Here's how the part is built. I have some questions about the finished solid (model axes, mm). Face numbers are marked on the shaded views. A direction names the side the tool comes from. Give positions to 0.01 mm unless a question says otherwise; leave off trailing zeros. Loops run counter-clockwise (first coordinate to the right, second up) from the corner with the lowest first, then second, coordinate; pieces in that order, holes last. Notation, with made-up numbers: (19, -7.5) - (78, -7.5) arc R7 ccw to (78, 1.5) - close; hole circle Ø2 at (81.25, 71.25). An arc over 180 degrees is marked (long way). Use a Markdown table: item, result.
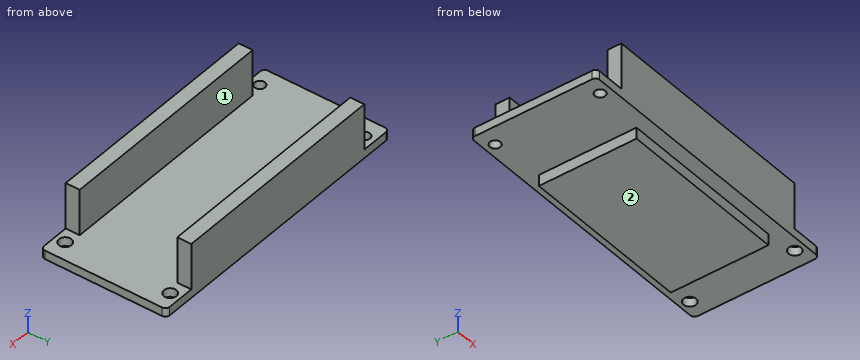
from build123d import *

# Parameters (mm, degrees)
SKETCH1_W           = 52.324
SKETCH1_H           = 22.86
BOSS_EXTRUDE1_DEPTH = 1.5748
SKETCH2_W           = 30.988
SKETCH2_H           = 17.78
BOSS_EXTRUDE2_DEPTH = 2.032
SKETCH3_W           = 40.64
SKETCH3_H           = 2.54
BOSS_EXTRUDE3_DEPTH = 8.382
FILLET1_R           = 0.762
SKETCH4_R           = 1.143
SKETCH4_R_2         = 0.9525
CUT_EXTRUDE1_DEPTH  = 1.5748


with BuildPart() as part:
    # Sketch1 → Boss-Extrude1 (new body)
    with BuildSketch(Plane.XY):
        with Locations((26.162, 11.43)):
            Rectangle(SKETCH1_W, SKETCH1_H)
    extrude(amount=BOSS_EXTRUDE1_DEPTH)

    # Sketch2 → Boss-Extrude2 (add)
    with BuildSketch(Plane(origin=(0, 0, 0), x_dir=(-1, 0, 0), z_dir=(0, 0, -1))):
        with Locations((-28.194, 11.43)):
            Rectangle(SKETCH2_W, SKETCH2_H)
    extrude(amount=BOSS_EXTRUDE2_DEPTH)

    # Sketch3 → Boss-Extrude3 (add)
    with BuildSketch(Plane.XY.offset(1.5748)):
        with Locations((26.162, 21.59)):
            Rectangle(SKETCH3_W, SKETCH3_H)
        with Locations((26.162, 1.27)):
            Rectangle(SKETCH3_W, SKETCH3_H)
    extrude(amount=BOSS_EXTRUDE3_DEPTH)

    # Fillet1
    fillet1_edges = [part.edges().sort_by_distance(p)[0] for p in [
        (0, 22.86, 0.7874),
        (52.324, 22.86, 0.7874),
        (52.324, 0, 0.7874),
        (0, 0, 0.7874),
    ]]
    fillet(fillet1_edges, radius=FILLET1_R)

    # Sketch4 → Cut-Extrude1 (cut)
    with BuildSketch(Plane(origin=(0, 0, 0), x_dir=(-1, 0, 0), z_dir=(0, 0, -1))):
        with Locations((-49.022, 20.9931)):
            Circle(SKETCH4_R)
        with Locations((-3.302, 20.9931)):
            Circle(SKETCH4_R_2)
        with Locations((-3.302, 1.8669)):
            Circle(SKETCH4_R_2)
        with Locations((-49.022, 1.8669)):
            Circle(SKETCH4_R)
    extrude(amount=-CUT_EXTRUDE1_DEPTH, mode=Mode.SUBTRACT)


solid = part.part
(1) If I drill on line 1 (X direction, y = 2, z = 1); line 2 (Y direction, x = 33, z = 4.5); line 3 (Z direction, x = 31, y = 8), over which ranges is the centre line in solid material (lowest first)?
A:
| item | result |
|---|---|
| line 1 | 0 to 2.36, 4.25 to 47.89, 50.16 to 52.32 |
| line 2 | 0 to 2.54, 20.32 to 22.86 |
| line 3 | -2.03 to 1.57 |
(2) Will these pins go through, and if not, where does the flat tip stop? pin 1 (0.8 mm diameter, centred on y = 21, z = 5.5, fed in from +X); pin 2 (2 mm diameter, centred on x = 3.3, y = 1.87, fed in from -Z); pin 3 (1.6 mm diameter, centred on y = 14, z = -1.5, fed in from +X); pin 4 (2.5 mm diameter, centred on x = 24.5, z = 7.5, fed in from -Y).
A:
| item | result |
|---|---|
| pin 1 | x = 46.48 |
| pin 2 | z = 0 |
| pin 3 | x = 43.69 |
| pin 4 | y = 0 |
(3) Suppose I cut it at D-D on x = 33.5. Write out the boundary of the cut face in (y, z), plus the area to 3 significant figures.
A:
| item | result |
|---|---|
| outline | (0, 0) - (2.54, 0) - (2.54, -2.03) - (20.32, -2.03) - (20.32, 0) - (22.86, 0) - (22.86, 9.96) - (20.32, 9.96) - (20.32, 1.57) - (2.54, 1.57) - (2.54, 9.96) - (0, 9.96) - close |
| area | 115 mm2 |
(4) On a 3-axis mill with a long thin cutter (end or side, diameter ignored), from which of +Z, -Z, +X, -X, +Y, -Y can I reach the whole of each face in a straight line? I mean the marked faces 1 and 2. Say none if no direction works.
A:
| item | result |
|---|---|
| face 1 | +Z, +X, -X |
| face 2 | -Z, +X, -X, +Y, -Y |
(5) Suppose I cut it at C-C on y = 16. Write out the boundary of the cut face in (x, z).
A:
| item | result |
|---|---|
| outline | (0, 0) - (12.7, 0) - (12.7, -2.03) - (43.69, -2.03) - (43.69, 0) - (52.32, 0) - (52.32, 1.57) - (0, 1.57) - close |
(6) Suppose I cut it at B-B on x = 49.5. Write out the boundary of the cut face in (y, z), plus the area to 3 significant figures.
A:
| item | result |
|---|---|
| outline | (0, 0) - (0.83, 0) - (0.83, 1.57) - (0, 1.57) - close; (2.91, 0) - (19.95, 0) - (19.95, 1.57) - (2.91, 1.57) - close; (22.03, 0) - (22.86, 0) - (22.86, 1.57) - (22.03, 1.57) - close |
| area | 29.5 mm2 |
(7) Suppose I cut it at A-A on z = 4.75. Write out the boundary of the cut face in (x, y), plus the area to 3 significant figures.
A:
| item | result |
|---|---|
| outline | (5.84, 0) - (46.48, 0) - (46.48, 2.54) - (5.84, 2.54) - close; (5.84, 20.32) - (46.48, 20.32) - (46.48, 22.86) - (5.84, 22.86) - close |
| area | 206 mm2 |
